Geometry: final body of the model. Coordinates: model frame, mm. Face numbers are marked on the shaded views. A direction names the side the tool comes from. Coordinates: 2 decimals unless noted, no trailing zeros. Order: outer loops, then holes, each group sorted by start corner. A loop starts at its lowest first (then second) coordinate and runs counter-clockwise, first axis right, second up. Notation, with made-up numbers: M 28,-7.75 L 84,-7.75 A37 cw 84,31.25 Z; hole C -3,19 d7. An arc over 180 degrees is marked long. Write item = value, one per line.
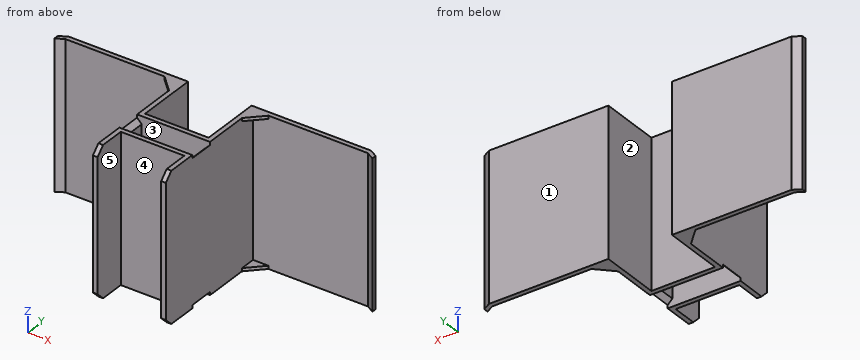
from build123d import *

# Parameters (mm, degrees)
SKETCH1_W                = 47
SKETCH1_H                = 42
BOSS_EXTRUDE1_DEPTH      = 95
SHELL1_T                 = -3
SKETCH2_W                = 95
SKETCH2_H                = 3
BOSS_EXTRUDE2_DEPTH      = 74
SKETCH3_W                = 3
SKETCH3_H                = 95
BOSS_EXTRUDE3_DEPTH      = 40
SKETCH4_W                = 95
SKETCH4_H                = 3
BOSS_EXTRUDE4_DEPTH      = 41
CHAMFER2_SIZE            = 5
CHAMFER3_SIZE            = 5
BOSS_EXTRUDE5_DEPTH      = 95
SKETCH10_W               = 10
SKETCH10_H               = 2
BOSS_EXTRUDE7_DEPTH      = 10
CHAMFER5_SIZE            = 10
CHAMFER5_OF_MIRROR5_SIZE = 10


# Some blends are built 0.0001 mm under size
with BuildPart() as part:
    # Sketch1 → Boss-Extrude1 (new body)
    with BuildSketch(Plane.XY):
        Rectangle(SKETCH1_W, SKETCH1_H)
    extrude(amount=BOSS_EXTRUDE1_DEPTH)

    # Shell1
    shell1_openings = [part.faces().sort_by_distance(p)[0] for p in [
        (0, 0, 95),
        (0, 0, 0),
        (0, 21, 47.5),
    ]]
    offset(amount=SHELL1_T, openings=shell1_openings, kind=Kind.INTERSECTION)

    # Sketch2 → Boss-Extrude2 (add)
    with BuildSketch(Plane.ZY.offset(23.5)):
        with Locations((47.5, 19.5)):
            Rectangle(SKETCH2_W, SKETCH2_H)
    boss_extrude2 = extrude(amount=BOSS_EXTRUDE2_DEPTH)

    # Mirror1: Boss-Extrude2 across plane
    add(boss_extrude2.mirror(Plane(origin=(0, 0, 0), x_dir=(0, 0, 1), z_dir=(1, 0, 0))))

    # Sketch3 → Boss-Extrude3 (add)
    with BuildSketch(Plane.XZ.offset(21)):
        with Locations((-22, 47.5)):
            Rectangle(SKETCH3_W, SKETCH3_H)
        with Locations((22, 47.5)):
            Rectangle(SKETCH3_W, SKETCH3_H)
    extrude(amount=BOSS_EXTRUDE3_DEPTH)

    # Sketch4 → Boss-Extrude4 (add)
    with BuildSketch(Plane.ZY.offset(-20.5)):
        with Locations((47.5, -38.5)):
            Rectangle(SKETCH4_W, SKETCH4_H)
    extrude(amount=BOSS_EXTRUDE4_DEPTH)

    # Chamfer2
    chamfer2_edges = [part.edges().sort_by_distance(p)[0] for p in [
        (-22, -61, 0),
        (-22, -61, 95),
        (22, -61, 95),
        (22, -61, 0),
    ]]
    chamfer(chamfer2_edges, length=CHAMFER2_SIZE)

    # Chamfer3
    # the kernel refuses this chamfer: 5 mm, written as the material it takes off along each edge
    with BuildSketch(Plane(origin=(-20.5, -21, 95), x_dir=(-0.9996219169112968, 0, 0.0274958766105877), z_dir=(0, -1, 0)), Plane(origin=(20.5, -21, 0), x_dir=(0.9996219169112968, 0, -0.027495876610586372), z_dir=(0, -1, 0))) as chamfer3_piece_1:
        Polygon((CHAMFER3_SIZE * 0.999621916911, CHAMFER3_SIZE * 0.0274958766106), (-CHAMFER3_SIZE * 0.0274958766106, CHAMFER3_SIZE * 0.999621916911), (0, 0), align=None)
    extrude(amount=16, mode=Mode.SUBTRACT)
    with BuildSketch(Plane(origin=(-20.5, -21, 0), x_dir=(-0.9996219169112968, 0, -0.027495876610586372), z_dir=(0, -1, 0)), Plane(origin=(20.5, -21, 95), x_dir=(0.9996219169112968, 0, 0.0274958766105877), z_dir=(0, -1, 0))) as chamfer3_piece_2:
        Polygon((CHAMFER3_SIZE * 0.999621916911, -CHAMFER3_SIZE * 0.0274958766106), (-CHAMFER3_SIZE * 0.0274958766106, -CHAMFER3_SIZE * 0.999621916911), (0, 0), align=None)
    extrude(amount=16, mode=Mode.SUBTRACT)

    # Sketch5 → Boss-Extrude5 (add)
    with BuildSketch(Plane(origin=(0, 0, 0), x_dir=(-1, 0, 0), z_dir=(0, 0, -1))):
        Polygon((97.5, 18), (97.5, 21), (102.5, 18.113248654), (102.5, 15.113248654), align=None)
    boss_extrude5 = extrude(amount=-BOSS_EXTRUDE5_DEPTH)

    # Mirror2: Boss-Extrude5 across plane
    add(boss_extrude5.mirror(Plane(origin=(0, 0, 0), x_dir=(0, 0, 1), z_dir=(1, 0, 0))))

    # Sketch10 → Boss-Extrude7 (add)
    with BuildSketch(Plane.XZ.offset(-18)):
        with Locations((-28.5, 94)):
            Rectangle(SKETCH10_W, SKETCH10_H)
        with Locations((-28.5, 1)):
            Rectangle(SKETCH10_W, SKETCH10_H)
    boss_extrude7 = extrude(amount=BOSS_EXTRUDE7_DEPTH)

    # Chamfer5
    chamfer5_edges = [part.edges().sort_by_distance(p)[0] for p in [
        (-33.5, 8, 94),
        (-33.5, 8, 1),
    ]]
    chamfer(chamfer5_edges, length=CHAMFER5_SIZE - 0.0001)  # a hair under: the kernel refuses the full size

    # Mirror5: Boss-Extrude7 across plane
    add(boss_extrude7.mirror(Plane(origin=(0, 0, 0), x_dir=(0, 0, 1), z_dir=(1, 0, 0))))

    # Chamfer5 of Mirror5
    chamfer5_of_mirror5_edges = [part.edges().sort_by_distance(p)[0] for p in [
        (33.5, 8, 94),
        (33.5, 8, 1),
    ]]
    chamfer(chamfer5_of_mirror5_edges, length=CHAMFER5_OF_MIRROR5_SIZE - 0.0001)  # a hair under: the kernel refuses the full size


solid = part.part
1) Mould query, pull axis Y, two halves, no side actions, for the marked faces 3, 4 and 5. Classes: pulls with the +Y half, pulls with the -Y half, needs draft (parallel to the pull), parting line crosses it, or undercut.
Numbers:
face_3 = undercut
face_4 = pulls with the -Y half
face_5 = needs draft
2) Section D-D, the plane x = -80.5. Return loops of the section in (y, z).
Numbers:
outline = M 18,0 L 21,0 L 21,95 L 18,95 Z
3) Set-up query: the marked faces 1 and 2. Return all of +Z, -Z, +X, -X, +Y, -Y with unobstructed straight access to the full face (end or side cutting, diameter ignored); none if empty.
Numbers:
face_1 = +Z, -Z, +X, -X, +Y
face_2 = +Z, -Z, +Y
4) Section A-A, the plane z = 9. Return loops of the section in (x, y), and give its area (3 significant figures).
Numbers:
outline = M -102.5,15.11 L -97.5,18 L -23.5,18 L -23.5,-61 L -20.5,-61 L -20.5,-40 L 20.5,-40 L 20.5,-61 L 23.5,-61 L 23.5,18 L 97.5,18 L 102.5,15.11 L 102.5,18.11 L 97.5,21 L 20.5,21 L 20.5,-18 L -20.5,-18 L -20.5,21 L -97.5,21 L -102.5,18.11 Z; hole M -20.5,-37 L 20.5,-37 L 20.5,-21 L -20.5,-21 Z
area = 1,210 mm²
5) Section B-B, the plane y = -34. Return loops of the section in (x, z).
Numbers:
outline = M -23.5,2 L -20.5,5 L -20.5,90 L -23.5,93 Z; M 20.5,5 L 23.5,2 L 23.5,93 L 20.5,90 Z
6) Pin query (flat end, axial travel): pin 1 (23.5 mm diameter, centred on y = -41, z = 42.5, fed in from +X); pin 2 (6 mm diameter, centred on x = -19, y = -26, fed in from +Z); pin 3 (10 mm diameter, centred on y = -44, z = 52, fed in from -X). Return the tip coordinate at first contact, or that it passes through.
Numbers:
pin_1 = 23.5
pin_2 = 91.5
pin_3 = -23.5
7) Line query: L1, parallel to X at y = -31.5, z = 61; L2, parallel to Y at x = -15.5, z = 86; L3, parallel to Y at x = 36, z = 91. Output: solid intervals per line, ascending.
Numbers:
L1 = -23.5 to -20.5, 20.5 to 23.5
L2 = -40 to -37, -21 to -18
L3 = 18 to 21
8) Section C-C, the plane x = -6. Return loops of the section in (y, z), and give its area (3 significant figures).
Numbers:
outline = M -40,0 L -37,0 L -37,95 L -40,95 Z; M -21,0 L -18,0 L -18,95 L -21,95 Z
area = 570 mm²
